For this review, take the finished solid that the model builds, in its own axes (mm). A direction names the side the tool comes from. Round coordinates to 2 decimals unless told otherwise and drop trailing zeros. Order: outer loops, then holes, each group sorted by start corner. A loop starts at its lowest first (then second) coordinate and runs counter-clockwise, first axis right, second up. Notation, with made-up numbers: (79.5, 76.5) -> (95.5, 76.5) arc R24 ccw to (95.5, 92.5) -> close; hole circle Ø6 at (-32, -31). An arc over 180 degrees is marked (long way). Answer in a Markdown table with one row per item.
```python
from build123d import *

# Parameters (mm, degrees)
SKETCH2_W           = 76.718161642
SKETCH2_H           = 53.12
BOSS_EXTRUDE1_DEPTH = 5
CUT_EXTRUDE1_DEPTH  = 10


with BuildPart() as part:
    # Sketch2 → Boss-Extrude1 (new body)
    with BuildSketch(Plane(origin=(0, 0, 0), x_dir=(-1, 0, 0), z_dir=(0, 0, -1))):
        with Locations((184.636580821, -28.44)):
            Rectangle(SKETCH2_W, SKETCH2_H)
    extrude(amount=BOSS_EXTRUDE1_DEPTH)

    # Sketch3 → Cut-Extrude1 (cut)
    with BuildSketch(Plane(origin=(0, 0, -5), x_dir=(-1, 0, 0), z_dir=(0, 0, -1))):
        Polygon((155.9375, -55), (155.9375, -51), (154.4875, -51), (154.4875, -48), (155.9375, -48), (155.9375, -42), (159.8375, -42), (159.8375, -48), (161.2875, -48), (161.2875, -51), (159.8375, -51), (159.8375, -55), align=None)
        Polygon((165.9375, -55), (165.9375, -51), (164.4875, -51), (164.4875, -48), (165.9375, -48), (165.9375, -42), (169.8375, -42), (169.8375, -48), (171.2875, -48), (171.2875, -51), (169.8375, -51), (169.8375, -55), align=None)
    extrude(amount=-CUT_EXTRUDE1_DEPTH, mode=Mode.SUBTRACT)


solid = part.part
```
Q1. Clearance check with a flat-ended pin moving along its axis: pin 1 Ø1.2 at (x, z) = (-168, -3.5) entering from -Y. State where the tip first meets the part, or that it passes through.
Answer key:
| item | result |
|---|---|
| pin 1 | stops at y = -42 |
Q2. Tool access review of faces 4 (the face through (-165, -48, -3)), 5 (the face through (-184, -28, -5)), 6 (the face through (-169.838, -45, -3)): name each direction out of +Z, -Z, +X, -X, +Y, -Y from which nothing blocks a thin tool from reaching the whole face with its end or side.
Answer key:
| item | result |
|---|---|
| face 4 | +Z, -Z |
| face 5 | -Z, +X, -X, +Y, -Y |
| face 6 | +Z, -Z, -Y |
Q3. Take a section at B-B, the plane z = -3.45. Write out the cut boundary in (x, y), then the cut area to 3 significant figures.
Answer key:
| item | result |
|---|---|
| outline | (-223, -55) -> (-169.84, -55) -> (-169.84, -51) -> (-171.29, -51) -> (-171.29, -48) -> (-169.84, -48) -> (-169.84, -42) -> (-165.94, -42) -> (-165.94, -48) -> (-164.49, -48) -> (-164.49, -51) -> (-165.94, -51) -> (-165.94, -55) -> (-159.84, -55) -> (-159.84, -51) -> (-161.29, -51) -> (-161.29, -48) -> (-159.84, -48) -> (-159.84, -42) -> (-155.94, -42) -> (-155.94, -48) -> (-154.49, -48) -> (-154.49, -51) -> (-155.94, -51) -> (-155.94, -55) -> (-146.28, -55) -> (-146.28, -1.88) -> (-223, -1.88) -> close |
| area | 3,960 mm^2 |
Q4. Take a section at A-A, the plane y = -44. Write out the cut boundary in (x, z).
Answer key:
| item | result |
|---|---|
| outline | (-223, -5) -> (-169.84, -5) -> (-169.84, 0) -> (-223, 0) -> close; (-165.94, -5) -> (-159.84, -5) -> (-159.84, 0) -> (-165.94, 0) -> close; (-155.94, -5) -> (-146.28, -5) -> (-146.28, 0) -> (-155.94, 0) -> close |
Q5. To check wall thickness, follow probe 1 along X at (y, z) = (-50.5, -2.75); probe 2 along X at (y, z) = (-43.5, -4.3); probe 3 along Y at (x, z) = (-157, -2.35). State the ranges of each line that lie inside material, in increasing order.
Answer key:
| item | result |
|---|---|
| probe 1 | x = -223 to -171.29, -164.49 to -161.29, -154.49 to -146.28 |
| probe 2 | x = -223 to -169.84, -165.94 to -159.84, -155.94 to -146.28 |
| probe 3 | y = -42 to -1.88 |
Q6. The part is to be moulded in two halves that separate along X. For faces 1 (the face through (-222.996, -29, -2)), 2 (the face through (-164.488, -50, -3)), 3 (the face through (-184, -28, 0)), say which applies: +X half, -X half, draft (parallel to the pull), parting line (faces both ways), or undercut.
Answer key:
| item | result |
|---|---|
| face 1 | -X half |
| face 2 | undercut |
| face 3 | draft |
